Read the model definition and answer for the solid it produces. Units are mm, in the model's axes. Round coordinates to 2 decimals unless told otherwise and drop trailing zeros. Loops run counter-clockwise (first coordinate to the right, second up) from the corner with the lowest first, then second, coordinate; pieces in that order, holes last. Notation, with made-up numbers: M -13.5,14 L -9.5,14 A27 ccw -9.5,49 Z; hole C 25.25,-2 d5. An arc over 180 degrees is marked long. Write each question's results on one line, items separated by ' | '.
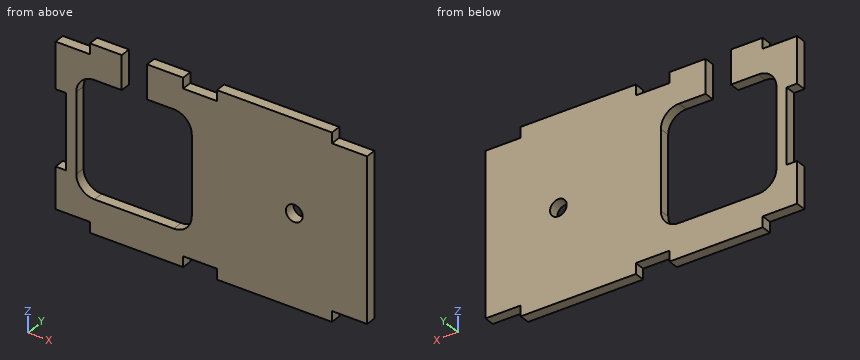
```python
from build123d import *

# Parameters (mm, degrees)
SKETCH1_W             = 172.72
SKETCH1_H             = 101.6
BOSS_EXTRUDE1_DEPTH   = 5.85
SKETCH5_R             = 4.635
CUT_EXTRUDE10_DEPTH   = 20
FILLET6_R             = 10
CAVITY1_START         = -50.8
CAVITY1_OUTLINE_W     = 19.066688648
CAVITY1_OUTLINE_H     = 5.85
CAVITY1_OUTLINE_W_2   = 18.685550926
CAVITY1_OUTLINE_W_3   = 19.50170991
CAVITY1_DEPTH         = 5.85
CAVITY1_START_2       = 44.95
CAVITY1_2_OUTLINE_W   = 19.066688648
CAVITY1_2_OUTLINE_H   = 5.85
CAVITY1_2_OUTLINE_W_2 = 18.685550926
CAVITY1_2_OUTLINE_W_3 = 19.50170991
CAVITY1_2_DEPTH       = 5.85
CAVITY1_START_3       = -22.02311963
CAVITY1_3_OUTLINE_W   = 5.85
CAVITY1_3_OUTLINE_H   = 5.85
CAVITY1_3_DEPTH       = 41.475447085


# Read off the part's stored shape, not the designer's step: Cavity1
with BuildPart() as part:
    # Sketch1 → Boss-Extrude1 (new body)
    with BuildSketch(Plane(origin=(0, 0, 0), x_dir=(1, 0, 0), z_dir=(0, 1, 0))):
        Rectangle(SKETCH1_W, SKETCH1_H)
    extrude(amount=BOSS_EXTRUDE1_DEPTH)

    # Sketch5 → Cut-Extrude10 (cut)
    with BuildSketch(Plane(origin=(0, 0, 0), x_dir=(1, 0, 0), z_dir=(0, 1, 0))):
        with Locations(Location((45.9739194, 0, 0), (0, 0, 90))):
            Circle(SKETCH5_R)
        Polygon((-10.850825335, 32), (-10.850825335, 0), (-10.850825335, -32), (-35.627924906, -32), (-35.627924906, -50.8), (-49.659575094, -50.8), (-49.659575094, -32), (-74.850825335, -32), (-74.850825335, 32), (-42.850825335, 32), align=None)
    extrude(amount=CUT_EXTRUDE10_DEPTH, mode=Mode.SUBTRACT)

    # Fillet6
    fillet6_edges = [part.edges().sort_by_distance(p)[0] for p in [
        (-10.850825335, 2.925, -32),
        (-74.850825335, 2.925, -32),
        (-74.850825335, 2.925, 32),
        (-10.850825335, 2.925, 32),
    ]]
    fillet(fillet6_edges, radius=FILLET6_R)

    # Cavity1 outline → Cavity1 (cut)
    with BuildSketch(Plane.XY.offset(CAVITY1_START)):
        with Locations((-76.826655676, 2.925)):
            Rectangle(CAVITY1_OUTLINE_W, CAVITY1_OUTLINE_H)
        with Locations((-6.281963463, 2.925)):
            Rectangle(CAVITY1_OUTLINE_W_2, CAVITY1_OUTLINE_H)
        with Locations((76.609145045, 2.925)):
            Rectangle(CAVITY1_OUTLINE_W_3, CAVITY1_OUTLINE_H)
    extrude(amount=CAVITY1_DEPTH, mode=Mode.SUBTRACT)

    # Cavity1 2 outline → Cavity1 2 (cut)
    with BuildSketch(Plane.XY.offset(CAVITY1_START_2)):
        with Locations((-76.826655676, 2.925)):
            Rectangle(CAVITY1_2_OUTLINE_W, CAVITY1_2_OUTLINE_H)
        with Locations((-6.281963463, 2.925)):
            Rectangle(CAVITY1_2_OUTLINE_W_2, CAVITY1_2_OUTLINE_H)
        with Locations((76.609145045, 2.925)):
            Rectangle(CAVITY1_2_OUTLINE_W_3, CAVITY1_2_OUTLINE_H)
    extrude(amount=CAVITY1_2_DEPTH, mode=Mode.SUBTRACT)

    # Cavity1 3 outline → Cavity1 3 (cut)
    with BuildSketch(Plane.XY.offset(CAVITY1_START_3)):
        with Locations((-83.435, 2.925)):
            Rectangle(CAVITY1_3_OUTLINE_W, CAVITY1_3_OUTLINE_H)
    extrude(amount=CAVITY1_3_DEPTH, mode=Mode.SUBTRACT)


solid = part.part
```
1. Find section B-B, the plane z = 0. Give the vertices of the cut face in (x, y), then the cut area to 3 significant figures.
Completed:
outline: M -80.51,0 L -74.85,0 L -74.85,5.85 L -80.51,5.85 Z; M -10.85,0 L 41.34,0 L 41.34,5.85 L -10.85,5.85 Z; M 50.61,0 L 86.36,0 L 86.36,5.85 L 50.61,5.85 Z | area: 548 mm2
2. Given P1, Ø3, axis at y = 1.5, z = 8, coming from the -X side; P2, Ø3, axis at y = 4, z = -47.5, coming from the -X side; P3, Ø1.8, axis at x = -80, y = 2.5, coming from the -Z side; P4, Ø2, axis at x = -9.5, z = -23.5, coming from the -Y side, each flat-ended and moving along its own axis, determine where each tip first touches the part or whether it passes through.
Completed:
P1: stops at x = -80.51 | P2: stops at x = -67.29 | P3: stops at z = -44.95 | P4: stops at y = 0
3. Find section A-A, the plane x = -54. Give the vertices of the cut face in (y, z).
Completed:
outline: M 0,-50.8 L 5.85,-50.8 L 5.85,-32 L 0,-32 Z; M 0,32 L 5.85,32 L 5.85,50.8 L 0,50.8 Z
4. Find section C-C, the plane z = 10.5. Give the vertices of the cut face in (x, y), then the cut area to 3 significant figures.
Completed:
outline: M -80.51,0 L -74.85,0 L -74.85,5.85 L -80.51,5.85 Z; M -10.85,0 L 86.36,0 L 86.36,5.85 L -10.85,5.85 Z | area: 602 mm2
5. Find the intervals of material crossed by L1, parallel to X at y = 0.55, z = -0.5; L2, parallel to X at y = 2.8, z = 0; L3, parallel to Z at x = -61.5, y = 2.9, in increasing order.
Completed:
L1: x = -80.51 to -74.85, -10.85 to 41.37, 50.58 to 86.36 | L2: x = -80.51 to -74.85, -10.85 to 41.34, 50.61 to 86.36 | L3: z = -50.8 to -32, 32 to 50.8
6. Find section D-D, the plane x = -6. Give the vertices of the cut face in (y, z), then the cut area to 3 significant figures.
Completed:
outline: M 0,-44.95 L 5.85,-44.95 L 5.85,44.95 L 0,44.95 Z | area: 526 mm2
